from build123d import *

# Parameters (mm, degrees)
SKETCH_1_W                = 680
SKETCH_1_H                = 480
EXTRUDE_1_DEPTH           = 20
FILLET_1_R                = 9
CHAMFER_3_SIZE            = 2
HOLE_WIZARD_M30_1_D       = 26.5
HOLE_WIZARD_M30_1_DEPTH   = 70.5
HOLE_WIZARD_M30_1_TIP     = 7.961403202
HOLE_WIZARD_1_D           = 9
HOLE_WIZARD_1_DEPTH       = 70.5
HOLE_WIZARD_1_CBORE_D     = 15
HOLE_WIZARD_1_CBORE_DEPTH = 9
HOLE_WIZARD_1_TIP         = 2.703872786
SKETCH_8_R                = 15
CUT_EXTRUDE_2_DEPTH       = 417.65333312
CHAMFER_5_SIZE            = 2
HOLE_WIZARD_M6_1_D        = 5
HOLE_WIZARD_M8_1_D        = 6.8
HOLE_WIZARD_2_D           = 6.6
HOLE_WIZARD_2_DEPTH       = 19.75
HOLE_WIZARD_2_CBORE_D     = 11
HOLE_WIZARD_2_CBORE_DEPTH = 6.8
HOLE_WIZARD_2_TIP         = 1.982840043


with BuildPart() as part:
    # 草图1 → 凸台-拉伸1 (new body)
    with BuildSketch(Plane.XY):
        Rectangle(SKETCH_1_W, SKETCH_1_H)
    extrude(amount=EXTRUDE_1_DEPTH)

    # 圆角1
    fillet_1_edges = [part.edges().sort_by_distance(p)[0] for p in [
        (340, -240, 10),
        (-340, -240, 10),
        (-340, 240, 10),
        (340, 240, 10),
    ]]
    fillet(fillet_1_edges, radius=FILLET_1_R)

    # 倒角3
    chamfer_3_edges = [part.edges().sort_by_distance(p)[0] for p in [
        (-340, 0, 0),
        (-340, 0, 20),
        (340, 0, 0),
        (0, -240, 0),
        (0, 240, 0),
        (-337.363961031, -237.363961031, 0),
        (337.363961031, -237.363961031, 0),
        (337.363961031, 237.363961031, 0),
        (-337.363961031, 237.363961031, 0),
        (0, 240, 20),
        (340, 0, 20),
        (0, -240, 20),
        (-337.363961031, -237.363961031, 20),
        (337.363961031, -237.363961031, 20),
        (337.363961031, 237.363961031, 20),
        (-337.363961031, 237.363961031, 20),
    ]]
    chamfer(chamfer_3_edges, length=CHAMFER_3_SIZE)

    # M30 螺纹孔1
    with Locations(Plane(origin=(0, 0, 0), x_dir=(-1, 0, 0), z_dir=(0, 0, -1))):
        with Locations((0, 210), (-310, 0), (0, -210), (310, 0)):
            Hole(HOLE_WIZARD_M30_1_D / 2, depth=HOLE_WIZARD_M30_1_DEPTH)
            with Locations((0, 0, -(HOLE_WIZARD_M30_1_DEPTH + HOLE_WIZARD_M30_1_TIP / 2))):  # 118° drill point
                Cone(0, HOLE_WIZARD_M30_1_D / 2, HOLE_WIZARD_M30_1_TIP, mode=Mode.SUBTRACT)

    # 打孔尺寸(%根据)内六角圆柱头螺钉的类型1
    with Locations(Plane(origin=(0, 0, 0), x_dir=(-1, 0, 0), z_dir=(0, 0, -1))):
        with Locations((20, -20), (-20, -20), (-20, 20), (20, 20)):
            CounterBoreHole(HOLE_WIZARD_1_D / 2, HOLE_WIZARD_1_CBORE_D / 2, HOLE_WIZARD_1_CBORE_DEPTH, depth=HOLE_WIZARD_1_DEPTH)
            with Locations((0, 0, -(HOLE_WIZARD_1_DEPTH + HOLE_WIZARD_1_TIP / 2))):  # 118° drill point
                Cone(0, HOLE_WIZARD_1_D / 2, HOLE_WIZARD_1_TIP, mode=Mode.SUBTRACT)

    # 草图8 → 切除-拉伸2 (cut, through all)
    with BuildSketch(Plane.XY.offset(20)):
        Circle(SKETCH_8_R)
    extrude(amount=-CUT_EXTRUDE_2_DEPTH, mode=Mode.SUBTRACT)

    # 倒角5
    chamfer_5_edges = [part.edges().sort_by_distance(p)[0] for p in [
        (-15, 0, 0),
        (-15, 0, 20),
    ]]
    chamfer(chamfer_5_edges, length=CHAMFER_5_SIZE)

    # M6 螺纹孔1 (through all)
    with Locations(Plane.XY.offset(20)):
        with Locations((65, -20), (20, 95), (20, 65), (-20, 65), (-20, 95), (20, -65), (20, -95), (-20, -95), (-20, -65), (-95, 20), (-65, 20), (-65, -20), (-95, -20), (65, 20), (95, 20), (95, -20)):
            Hole(HOLE_WIZARD_M6_1_D / 2)

    # M8 螺纹孔1 (through all)
    with Locations(Plane(origin=(0, 0, 0), x_dir=(-1, 0, 0), z_dir=(0, 0, -1))):
        with Locations((330.25, -231.25), (285.75, -231.25), (285.75, -156.75), (330.25, -156.75), (-285.75, -231.25), (-330.25, -231.25), (-330.25, -156.75), (-285.75, -156.75), (330.25, 156.75), (285.75, 156.75), (285.75, 231.25), (330.25, 231.25), (-285.75, 156.75), (-330.25, 156.75), (-330.25, 231.25), (-285.75, 231.25)):
            Hole(HOLE_WIZARD_M8_1_D / 2)

    # 打孔尺寸(%根据)内六角圆柱头螺钉的类型2
    with Locations(Plane(origin=(0, 0, 0), x_dir=(-1, 0, 0), z_dir=(0, 0, -1))):
        with Locations((225, -210), (75, -210), (-75, -210), (-225, -210), (225, 210), (75, 210), (-75, 210), (-225, 210), (310, -175), (310, 175), (-310, -175), (-310, 175), (-310, -75), (-310, 75), (310, -75), (310, 75)):
            CounterBoreHole(HOLE_WIZARD_2_D / 2, HOLE_WIZARD_2_CBORE_D / 2, HOLE_WIZARD_2_CBORE_DEPTH, depth=HOLE_WIZARD_2_DEPTH)
            with Locations((0, 0, -(HOLE_WIZARD_2_DEPTH + HOLE_WIZARD_2_TIP / 2))):  # 118° drill point
                Cone(0, HOLE_WIZARD_2_D / 2, HOLE_WIZARD_2_TIP, mode=Mode.SUBTRACT)


solid = part.part
Work out the finished part from the listing and answer in its coordinate system (mm). A direction names the side the tool comes from. Give positions to 0.01 mm unless a question says otherwise; leave off trailing zeros. Answer in a Markdown table with one row per item. Add a question column.
Q1. Each of these flat-tipped pins is pushed along its axis until it touches: P1, Ø3, axis at x = 65, y = -20, coming from the -Z side; P2, Ø10.5, axis at x = 225, y = -210, coming from the -Z side. Where does it stop, or does it pass through?
Q2. A tool of negligible diameter and unlimited length cuts with its end or side. For faces 4 (the cylindrical face through (-12.507, -19.67, 4.437)), 5 (the flat face through (-5, 240, 10)), from which of +Z, -Z, +X, -X, +Y, -Y can it reach the whole face along a straight path? Write none if from no direction.
Q3. Determine the mould class of faces 1 (the cylindrical face through (-14.985, 0.66, 10.112)), 2 (the flat face through (-5, -240, 10)), 3 (the flat face through (-340, -3, 10)) for opening direction Y: released by +Y, released by -Y, zero draft, split by the parting line, or undercut.
Q4. Consider line 1 along X through (y, z) = (156.75, 11.75); line 2 along Y through (x, z) = (95, 11); line 3 along X through (y, z) = (-209, 12.5). Determine where each line is inside the solid, lowest interval first.
Solution:
| question | item | result |
|---|---|---|
| 1 | P1 | passes through |
| 1 | P2 | stops at z = 6.8 |
| 2 | face 4 | -Z |
| 2 | face 5 | +Z, -Z, +X, -X, +Y |
| 3 | face 1 | undercut |
| 3 | face 2 | released by -Y |
| 3 | face 3 | zero draft |
| 4 | line 1 | x = -340 to -333.65, -326.85 to -289.15, -282.35 to 282.35, 289.15 to 326.85, 333.65 to 340 |
| 4 | line 2 | y = -240 to -22.5, -17.5 to 17.5, 22.5 to 240 |
| 4 | line 3 | x = -340 to -228.14, -221.86 to -78.14, -71.86 to -13.21, 13.21 to 71.86, 78.14 to 221.86, 228.14 to 340 |
